from build123d import *

# Parameters (mm, degrees)
ESQUISSE1_W             = 10
ESQUISSE1_H             = 5
BOSS_EXTRU_1_DEPTH      = 5
ENL_V_MAT_EXTRU_1_DEPTH = 307.896155075


with BuildPart() as part:
    # Esquisse1 → Boss.-Extru.1 (new body)
    with BuildSketch(Plane.XY):
        with BuildLine():
            Line((0, 0), (43, 0))
            Line((43, 0), (43, -20.443064708))
            Line((43, -20.443064708), (48, -20.443064708))
            Line((48, -20.443064708), (53.856481481, -77.64404044))
            Line((53.856481481, -77.64404044), (48.882483592, -78.153299699))
            Line((48.882483592, -78.153299699), (50.919520629, -98.049291258))
            Line((50.919520629, -98.049291258), (55.893518519, -97.540031998))
            Line((55.893518519, -97.540031998), (61.75, -154.74100773))
            Line((61.75, -154.74100773), (56.77600211, -155.250266989))
            Line((56.77600211, -155.250266989), (58.813039147, -175.146258548))
            Line((58.813039147, -175.146258548), (63.787037037, -174.636999289))
            Line((63.787037037, -174.636999289), (64.5, -181.600596335))
            Line((64.5, -181.600596335), (24.488887394, -288.882285677))
            ThreePointArc((24.488887394, -288.882285677), (19.131421435, -296.900300104), (10, -300))
            Line((10, -300), (-5, -300))
            Line((-5, -300), (-5, -280))
            Line((-5, -280), (0, -280))
            Line((0, -280), (0, -250))
            Line((0, -250), (-5, -250))
            Line((-5, -250), (-5, -230))
            Line((-5, -230), (0, -230))
            Line((0, -230), (0, -210))
            Line((0, -210), (-5, -210))
            Line((-5, -210), (-5, -160))
            Line((-5, -160), (0, -160))
            Line((0, -160), (0, -140))
            Line((0, -140), (-5, -140))
            Line((-5, -140), (-5, -90))
            Line((-5, -90), (0, -90))
            Line((0, -90), (0, -70))
            Line((0, -70), (-5, -70))
            Line((-5, -70), (-5, -20))
            Line((-5, -20), (0, -20))
            Line((0, -20), (0, 0))
        make_face()
        with Locations((24.5, -138.5)):
            Rectangle(ESQUISSE1_W, ESQUISSE1_H, mode=Mode.SUBTRACT)
        Polygon((11.000546858, -23.352307985), (4.424979656, -36.83421868), (8.918949887, -39.026074414), (15.494517089, -25.544163719), align=None, mode=Mode.SUBTRACT)
    extrude(amount=BOSS_EXTRU_1_DEPTH)

    # Esquisse3 → Enlèv. mat.-Extru.1 (cut, through all)
    with BuildSketch(Plane(origin=(0, 0, 0), x_dir=(-1, 0, 0), z_dir=(0, 0, -1))):
        Polygon((-43, -20.443064708), (-40.91621031, 0), (-43, 0), align=None)
    extrude(amount=-ENL_V_MAT_EXTRU_1_DEPTH, mode=Mode.SUBTRACT)


solid = part.part
Geometry: final body of the model. Coordinates: model frame, mm. A direction names the side the tool comes from. Round coordinates to 2 decimals unless told otherwise and drop trailing zeros. Loops run counter-clockwise (first coordinate to the right, second up) from the corner with the lowest first, then second, coordinate; pieces in that order, holes last.
Q1. Access query for faces 5 (the flat face through (-5, -240, 2)), 6 (the flat face through (59.3, -154.99, 2.46)), 7 (the flat face through (0, -150, 2)), 8 (the flat face through (53.37, -97.8, 2.46)), 9 (the flat face through (-3, -20, 2)). Directions: +Z, -Z, +X, -X, +Y, -Y. A direction counts if a zero-diameter tool reaches every point of the face in a straight line with its end or side. Return the directions, or none.
Q2. Section C-C on x = 33. Return loops of the section in (y, z), plus the area to 3 significant figures.
Q3. Material intervals for L1, parallel to Y at x = 23.5, z = 3.05; L2, parallel to Y at x = 14.5, z = 4.35; L3, parallel to X at y = -26.5, z = 3, sorted ascending.
Q4. Pin query (flat end, axial travel): P1, Ø2.5, axis at y = -261.5, z = 2, coming from the -X side; P2, Ø2.5, axis at x = -3, z = 2, coming from the +Y side. Return the tip coordinate at first contact, or that it passes through.
Q5. Section A-A on z = 3.75. State how many separate pieces and enclosed holes the cut face has, plus the area to 3 significant figures.
Q6. Section B-B on y = -125.5. Return loops of the section in (x, z).
Q7. Pull-direction query (Y, two-part tool) for faces 1 (the flat face through (-3, -230, 2)), 2 (the flat face through (50.887, -48.643, 2.465)), 3 (the flat face through (51.404, -77.895, 2.465)), 4 (the flat face through (23, -148, 5)); classes: released by +Y, released by -Y, zero draft, split by the parting line, or undercut.
Evaluation:
1. face 5: +Z, -Z, -X, +Y, -Y
1. face 6: +Z, -Z, +X
1. face 7: +Z, -Z, -X
1. face 8: +Z, -Z
1. face 9: +Z, -Z, -X, +Y
2. outline: (-266.06, 0) - (0, 0) - (0, 5) - (-266.06, 5) - close
2. area: 1,330 mm2
3. L1: y = -291.54 to -141, -136 to 0
3. L2: y = -299.31 to -27.58, -25.06 to 0
3. L3: x = -5 to 9.47, 15.03 to 48.62
4. P1: stops at x = 0
4. P2: stops at y = -20
5. separate pieces: 1
5. enclosed holes: 2
5. area: 15,600 mm2
6. outline: (-5, 0) - (58.76, 0) - (58.76, 5) - (-5, 5) - close
7. face 1: undercut
7. face 2: released by +Y
7. face 3: undercut
7. face 4: zero draft
